Autodesk Inventor part; units mm, degrees
ref_plane "YZ Plane" through (0, 0, 0) normal (1, 0, 0) x (0, 1, 0)
ref_plane "XZ Plane" through (0, 0, 0) normal (0, 1, 0) x (-1, 0, 0)
ref_plane "XY Plane" through (0, 0, 0) normal (0, 0, 1) x (1, 0, 0)
sketch "Sketch1" plane through (0, 0, 0) normal (0, 1, 0) x (-1, 0, 0)
  line L0 (0, 0) -> (30, 0)
  line L1 (30, 0) -> (30, -34)
  line L2 (30, -34) -> (0, -34)
  line L3 (0, -34) -> (0, 0)
  dimension "d0" = 30
  dimension "d1" = 34
extrude "Extrusion1" add sketch "Sketch1" along normal blind 25
sketch "Sketch2" plane through (0, 0, 0) normal (1, 0, 0) x (0, 0, -1)
  line L0 (34, 0) -> (0, 0)
  line L1 (17, 0) -> (17, 25) construction
  line L2 (34, 25) -> (0, 25)
  circle A0 centre (17, 12) radius 5.25
  circle A1 centre (17, 12) radius 10.2956 construction
  dimension "d4" = 10.5
  dimension "d5" = 12
extrude "Extrusion2" cut sketch "Sketch2" against normal blind 30
sketch "Sketch3" plane through (0, 0, 0) normal (1, 0, 0) x (0, 0, -1)
  circle A0 centre (17, 12) radius 5.25
  circle A1 centre (17, 12) radius 8 construction
  circle A2 centre (17, 20) radius 1.6
  point P0 (0, 0)
  dimension "d8" = 16
  dimension "d9" = 3.2
extrude "Extrusion3" cut sketch "Sketch3" against normal blind 30 contours A2
pattern_circular "Circular Pattern1" count 4 over 360 about axis through (0, 12, -17) along (-1, 0, 0) of "Extrusion3"
sketch "Sketch4" plane through (0, 25, 0) normal (0, 1, 0) x (1, 0, 0)
  line L0 (0, 0) -> (0, 34)
  line L1 (0, 17) -> (-30, 17) construction
  line L2 (-30, 34) -> (-30, 0)
  line L3 (-5, 4.5) -> (-25, 4.5) construction
  line L4 (-25, 4.5) -> (-25, 29.5) construction
  line L5 (-25, 29.5) -> (-5, 29.5) construction
  line L6 (-5, 29.5) -> (-5, 4.5) construction
  line L7 (-5, 4.5) -> (-25, 29.5) construction
  line L8 (-25, 4.5) -> (-5, 29.5) construction
  circle A0 centre (-25, 4.5) radius 1.55
  circle A1 centre (-25, 29.5) radius 1.55
  circle A2 centre (-5, 29.5) radius 1.55
  circle A3 centre (-5, 4.5) radius 1.55
  point P0 (-15, 17)
  dimension "d15" = 20
  dimension "d16" = 25
  dimension "d17" = 3.1
  dimension "d18" = 3.1
  dimension "d19" = 3.1
  dimension "d20" = 3.1
extrude "Extrusion4" cut sketch "Sketch4" against normal blind 30
fillet "Fillet2" radius 15 2 edges at (-15, 25, -34) (-15, 25, 0)
sketch "Sketch7" plane through (0, 25, 0) normal (0, 1, 0) x (1, 0, 0)
  circle A0 centre (-25, 4.5) radius 1.55
  circle A1 centre (-25, 4.5) radius 3
  circle A2 centre (-25, 29.5) radius 1.55
  circle A3 centre (-25, 29.5) radius 3
  circle A4 centre (-5, 29.5) radius 1.55
  circle A5 centre (-5, 29.5) radius 3
  circle A6 centre (-5, 4.5) radius 1.55
  circle A7 centre (-5, 4.5) radius 3
  point P0 (0, 0)
  dimension "d46" = 6
  dimension "d47" = 6
  dimension "d48" = 6
  dimension "d49" = 6
extrude "Extrusion7" cut sketch "Sketch7" against normal blind 11 contours A0 | A1 | A2 | A3 | A4 | A5 | A6 | A7
properties part number "Nut holder"
Geometry: final body of the model. Coordinates: model frame, mm. A direction names the side the tool comes from. Coordinates: 2 decimals unless noted, no trailing zeros. Order: outer loops, then holes, each group sorted by start corner. A loop starts at its lowest first (then second) coordinate and runs counter-clockwise, first axis right, second up. Notation, with made-up numbers: (-5.5, 64) -> (13.5, 64) arc R19 ccw to (13.5, 97) -> close; hole circle Ø4 at (9, -27). An arc over 180 degrees is marked (long way). Write each question's results on one line, items separated by ' | '. Start each with the question number.
1) Cut plane C-C, the plane z = -26. Output: boundary loops of the cut face in (x, y).
2) Material intervals for line 1 along X through (y, z) = (9.25, -4.5); line 2 along X through (y, z) = (17.75, -29.5); line 3 along Z through (x, y) = (-25, 3.5), sorted ascending.
3) Mould query, pull axis Z, two halves, no side actions, for faces 3 (the flat face through (-30, 7, -13)), 4 (the flat face through (-15, 5, -34)), 5 (the cylindrical face through (-14.79, 12.231, -11.755)). Classes: released by +Z, released by -Z, zero draft, split by the parting line, or undercut.
4) First-contact query: pin 1 (3 mm diameter, centred on x = -25, z = -29.5, fed in from -Y); pin 2 (3 mm diameter, centred on x = -6, z = -30, fed in from +Y); pin 3 (5 mm diameter, centred on x = -6, z = -3.5, fed in from +Y); pin 4 (1.5 mm diameter, centred on x = -10.5, y = 22.5, fed in from -Z). Flat tips, straight axial feed; report the tip coordinate or a pass-through.
5) Cut plane D-D, the plane x = -9. Output: boundary loops of the cut face in (y, z).
6) Cut plane A-A, the plane y = 4. Output: boundary loops of the cut face in (x, z), and give its area (3 significant figures).
7) Cut plane B-B, the plane x = -25. Output: boundary loops of the cut face in (y, z), and give its area (3 significant figures).
8) Set-up query: faces 1 (the flat face through (-15, 0, -17)), 2 (the flat face through (-24, 14, -28)). Return all of +Z, -Z, +X, -X, +Y, -Y with unobstructed straight access to the full face (end or side cutting, diameter ignored); none if empty.
Checks:
1) outline: (-30, 0) -> (0, 0) -> (0, 10.75) -> (-30, 10.75) -> close; (-30, 13.25) -> (0, 13.25) -> (0, 23.27) -> (-30, 23.27) -> close
2) line 1: -30 to -26.55, -23.45 to -6.55, -3.45 to 0 | line 2: -30 to -28, -22 to -8, -2 to 0 | line 3: -34 to -31.05, -27.95 to -18.52, -15.48 to -6.05, -2.95 to 0
3) face 3: zero draft | face 4: released by -Z | face 5: undercut
4) pin 1: through | pin 2: y = 14 | pin 3: y = 21.24 | pin 4: z = -28.32
5) outline: (0, -34) -> (10, -34) arc R15 ccw to (25, -19) -> (25, -15) arc R15 ccw to (10, 0) -> (0, 0) -> close; hole circle Ø3.2 at (4, -17); hole circle Ø10.5 at (12, -17); hole circle Ø3.2 at (12, -25); hole circle Ø3.2 at (12, -9); hole circle Ø3.2 at (20, -17)
6) outline: (-30, -34) -> (0, -34) -> (0, -18.6) -> (-30, -18.6) -> close; (-30, -15.4) -> (0, -15.4) -> (0, 0) -> (-30, 0) -> close; hole circle Ø3.1 at (-25, -29.5); hole circle Ø3.1 at (-25, -4.5); hole circle Ø3.1 at (-5, -29.5); hole circle Ø3.1 at (-5, -4.5) | area: 894 mm^2
7) outline: (0, -34) -> (10, -34) arc R15 ccw to (16.54, -32.5) -> (14, -32.5) -> (14, -31.05) -> (0, -31.05) -> close; (0, -27.95) -> (14, -27.95) -> (14, -26.5) -> (22.99, -26.5) arc R15 ccw to (25, -19) -> (25, -15) arc R15 ccw to (22.99, -7.5) -> (14, -7.5) -> (14, -6.05) -> (0, -6.05) -> close; (0, -2.95) -> (14, -2.95) -> (14, -1.5) -> (16.54, -1.5) arc R15 ccw to (10, 0) -> (0, 0) -> close; hole circle Ø3.2 at (4, -17); hole circle Ø10.5 at (12, -17); hole circle Ø3.2 at (12, -25); hole circle Ø3.2 at (12, -9); hole circle Ø3.2 at (20, -17) | area: 471 mm^2
8) face 1: +Z, -Z, +X, -X, -Y | face 2: +Y
